CAD build for the part. Positions are in the model's coordinates, mm. Coordinates: 2 decimals unless noted, no trailing zeros. Order: outer loops, then holes, each group sorted by start corner. A loop starts at its lowest first (then second) coordinate and runs counter-clockwise, first axis right, second up. Notation, with made-up numbers: M 39,59 L 92,59 A4 cw 92,64 Z; hole C 48.25,43 d11. An arc over 180 degrees is marked long. Write item = value, one per line. Start each with the question number.
Autodesk Inventor part; units mm, degrees
ref_plane "YZ Plane" through (0, 0, 0) normal (1, 0, 0) x (0, 1, 0)
ref_plane "XZ Plane" through (0, 0, 0) normal (0, 1, 0) x (-1, 0, 0)
ref_plane "XY Plane" through (0, 0, 0) normal (0, 0, 1) x (1, 0, 0)
sketch "main" plane through (0, 0, 0) normal (0, 0, 1) x (1, 0, 0)
  circle A0 centre (-6.1105, -12.0036) radius 2.1844
  circle A1 centre (-31.5105, -12.0036) radius 2.1844
  circle A2 centre (15.0202, -6.3416) radius 2.1844
  circle A3 centre (37.0172, 6.3584) radius 2.1844
  arc A4 (-31.5236, -5.6536) -> (-31.5105, -18.3536) centre (-31.5105, -12.0036) ccw
  arc A5 (40.1922, 0.8591) -> (33.8536, 11.8642) centre (37.0172, 6.3584) ccw
  arc A6 (-31.5236, -5.6536) -> (33.8536, 11.8642) centre (-31.796, 126.1175) ccw
  line L0 (-31.5105, -18.3536) -> (5.2134, -18.3536)
  line L1 (40.1922, 0.8591) -> (8.3884, -17.5028)
  circle A7 centre (5.2134, -12.0036) radius 2.0955
  arc A8 (5.2134, -18.3536) -> (8.3884, -17.5028) centre (5.2134, -12.0036) ccw
  line L2 (5.2134, -12.0036) -> (43.3134, -12.0036) construction
  point P0 (-0.7926, -1.6009)
  dimension "d0" = 12.7
  dimension "d3" = 12.7
  dimension "d7" = 4.191
  dimension "d8" = 6.35
  dimension "d13" = 25.4
sketch "Sketch1" plane through (0, 0, 0) normal (0, 0, 1) x (1, 0, 0)
  circle A0 centre (25.4, 0) radius 2.1844
  circle A1 centre (0, 0) radius 2.1844
  circle A2 centre (46.5307, 5.662) radius 2.1844
  circle A3 centre (68.5277, 18.362) radius 2.1844
  arc A4 (-0.0131, 6.35) -> (0, -6.35) centre (0, 0) ccw
  arc A5 (71.7027, 12.8627) -> (65.3641, 23.8678) centre (68.5277, 18.362) ccw
  arc A6 (-0.0131, 6.35) -> (65.3641, 23.8678) centre (-0.2855, 138.1211) ccw
  line L0 (0, -6.35) -> (36.7239, -6.35)
  line L1 (71.7027, 12.8627) -> (39.8989, -5.4993)
  circle A7 centre (36.7239, 0) radius 2.0955
  arc A8 (36.7239, -6.35) -> (39.8989, -5.4993) centre (36.7239, 0) ccw
  line L2 (36.7239, 0) -> (74.8239, 0) construction
extrude "Extrusion1" add sketch "Sketch1" along normal blind 1.5875
properties part number "60 Degree Gusset" material "Acetal Resin, White"
1. Slice it at B-B (y = 0). Write the cut outline in (x, z), plus the area to 3 significant figures.
2. Slice it at A-A (x = 1). Write the cut outline in (y, z).
3. Slice it at C-C (z = 0.4). Write the cut outline in (x, y), plus the area to 3 significant figures.
4. Flat gauge pin, fed straight in: pin 1 (3.5 mm diameter, centred on x = 68.53, y = 18.36, fed in from -Z). Where does the tip first touch, or does it go through?
5. Slice it at D-D (x = 36). Write the cut outline in (y, z), plus the area to 3 significant figures.
6. Probe L1, parallel to Y at x = 0, z = 1.05; L2, parallel to X at y = 17, z = 1.4; L3, parallel to Y at x = 25.4, z = 0.9. List the from-to ranges inside material, lowest first.
7. Mould opens along X. For faces 1 (the flat face through (34, 6, 1.588)), 2 (the cylindrical face through (38.39, -6.128, 0.783)), 3 (the cylindrical face through (73.96, 21.65, 0.78)), 4 (the cylindrical face through (66.8, 19.7, 0.8)) say: released by +X, released by -X, zero draft, split by the parting line, or undercut.
Calculated:
q1.outline = M -6.35,0 L -2.18,0 L -2.18,1.59 L -6.35,1.59 Z; M 2.18,0 L 23.22,0 L 23.22,1.59 L 2.18,1.59 Z; M 27.58,0 L 34.63,0 L 34.63,1.59 L 27.58,1.59 Z; M 38.82,0 L 49.42,0 L 49.42,1.59 L 38.82,1.59 Z
q1.area = 68.0 mm²
q2.outline = M -6.35,0 L -1.94,0 L -1.94,1.59 L -6.35,1.59 Z; M 1.94,0 L 6.36,0 L 6.36,1.59 L 1.94,1.59 Z
q3.outline = M -0.01,6.35 A6.35 ccw 0,-6.35 L 36.72,-6.35 A6.35 ccw 39.9,-5.5 L 71.7,12.86 A6.35 ccw 65.36,23.87 A131.77 cw Z; hole C 0,0 d4.37; hole C 25.4,0 d4.37; hole C 36.72,0 d4.19; hole C 46.53,5.66 d4.37; hole C 68.53,18.36 d4.37
q3.area = 1,090 mm²
q4.pin_1 = through
q5.outline = M -6.35,0 L -1.97,0 L -1.97,1.59 L -6.35,1.59 Z; M 1.97,0 L 11.44,0 L 11.44,1.59 L 1.97,1.59 Z
q5.area = 22.0 mm²
q6.L1 = -6.35 to -2.18, 2.18 to 6.35
q6.L2 = 51.61 to 66.82, 70.24 to 74.73
q6.L3 = -6.35 to -2.18, 2.18 to 8.88
q7.face_1 = zero draft
q7.face_2 = released by +X
q7.face_3 = split by the parting line
q7.face_4 = undercut
